from build123d import *

# Parameters (mm, degrees)
Y_KSEKLIK_EKSTR_ZYON1_DEPTH = 12
KES_EKSTR_ZYON1_DEPTH       = 10
KES_EKSTR_ZYON4_DEPTH       = 20
IZIM4_W                     = 6
IZIM4_H                     = 12
Y_KSEKLIK_EKSTR_ZYON2_DEPTH = 30
IZIM5_R                     = 2
KES_EKSTR_ZYON5_DEPTH       = 60


with BuildPart() as part:
    # Çizim1 → Yükseklik-Ekstrüzyon1 (new body)
    with BuildSketch(Plane.XY):
        with BuildLine():
            Line((-2.88077248, -55), (82.297274127, -55))
            ThreePointArc((82.297274127, -55), (131.991875204, 23.567915135), (39.708250823, 34.801940953))
            ThreePointArc((39.708250823, 34.801940953), (-52.575373557, 23.567915135), (-2.88077248, -55))
        make_face()
    extrude(amount=Y_KSEKLIK_EKSTR_ZYON1_DEPTH)

    # Çizim2 → Kes-Ekstrüzyon1 (cut, symmetric)
    with BuildSketch(Plane.XY):
        with BuildLine():
            Line((82.297274127, -53.5), (-2.88077248, -53.5))
            ThreePointArc((-2.88077248, -53.5), (-50.81065631, 23.769228763), (39.708250823, 32.379393047))
            ThreePointArc((39.708250823, 32.379393047), (130.227157957, 23.769228763), (82.297274127, -53.5))
        make_face()
    extrude(amount=KES_EKSTR_ZYON1_DEPTH, both=True, mode=Mode.SUBTRACT)

    # Çizim3 → Kes-Ekstrüzyon4 (cut)
    with BuildSketch(Plane.XZ.offset(55)):
        with BuildLine():
            Line((25.295548254, 4.99642351), (25.295548254, 0))
            Line((25.295548254, 0), (33.431042786, 0))
            Line((33.431042786, 0), (33.431042786, 4.99642351))
            ThreePointArc((33.431042786, 4.99642351), (29.36329552, 9.064170776), (25.295548254, 4.99642351))
        make_face()
        with BuildLine():
            Line((35.422473694, 4.99642351), (35.422473694, 0))
            Line((35.422473694, 0), (43.422473694, 0))
            Line((43.422473694, 0), (43.422473694, 4.99642351))
            ThreePointArc((43.422473694, 4.99642351), (39.422473694, 8.99642351), (35.422473694, 4.99642351))
        make_face()
        with BuildLine():
            Line((45.619413975, 4.99642351), (45.619413975, 0))
            Line((45.619413975, 0), (53.887629124, 0))
            Line((53.887629124, 0), (53.887629124, 4.99642351))
            ThreePointArc((53.887629124, 4.99642351), (49.753521549, 9.130531084), (45.619413975, 4.99642351))
        make_face()
    extrude(amount=-KES_EKSTR_ZYON4_DEPTH, mode=Mode.SUBTRACT)

    # Çizim4 → Yükseklik-Ekstrüzyon2 (add)
    with BuildSketch(Plane(origin=(0, -55, 0), x_dir=(-1, 0, 0), z_dir=(0, -1, 0))):
        with Locations((-17.243778266, -6)):
            Rectangle(IZIM4_W, IZIM4_H)
        with Locations((-61.695384492, -6)):
            Rectangle(IZIM4_W, IZIM4_H)
    extrude(amount=Y_KSEKLIK_EKSTR_ZYON2_DEPTH)

    # Çizim5 → Kes-Ekstrüzyon5 (cut)
    with BuildSketch(Plane(origin=(64.695384492, 0, 0), x_dir=(0, 0, -1), z_dir=(1, 0, 0))):
        with Locations(Location((-6, -81.004647187, 0), (0, 0, 90))):
            Circle(IZIM5_R)
    extrude(amount=-KES_EKSTR_ZYON5_DEPTH, mode=Mode.SUBTRACT)


solid = part.part
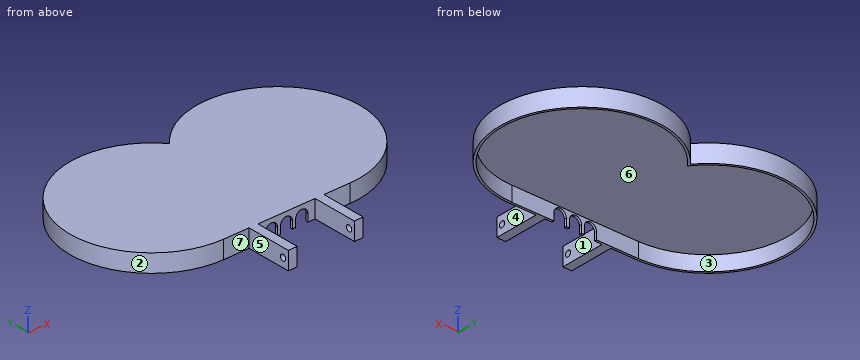
Can you work these out from the model? Positions are in its coordinate system, mm. Face numbers are marked on the shaded views. A direction names the side the tool comes from. Coordinates: 2 decimals unless noted, no trailing zeros. Write each loop counter-clockwise with the first axis right and the second up, starting at its lowest first coordinate (ties: lowest second). Pieces come first, ordered by that corner, then holes. Notation, with made-up numbers: (-36.5, 54.5) -> (-29.5, 54.5) arc R29 cw to (-29.5, 80.5) -> close; hole circle Ø8 at (68, 67.25). An arc over 180 degrees is marked (long way). Write each question's results on one line, items separated by ' | '. Start each with the question number.
Item 1: On a 3-axis mill with a long thin cutter (end or side, diameter ignored), from which of +Z, -Z, +X, -X, +Y, -Y can I reach the whole of each face in a straight line? I mean the marked faces 1, 2 and 3. Say none if no direction works.
Item 2: If we section it at B-B, the plane x = 116.5: Write out the boundary of the cut face in (y, z), and give its area (3 significant figures).
Item 3: Please list where these lines run through material, in increasing order: probe 1 along X at (y, z) = (-56, 1); probe 2 along X at (y, z) = (2, 5.75); probe 3 along X at (y, z) = (40.5, 3.25).
Item 4: Thinking about a two-plate mould opening in X: for the marked faces 4, 5, 6 and 7, which applies, released by +X, released by -X, zero draft, split by the parting line, or undercut?
Item 5: I'm going to push flat-ended pins straight in: P1, Ø5, axis at y = -62, z = 10, coming from the -X side; P2, Ø5, axis at x = 36, z = 6, coming from the +Y side; P3, Ø4, axis at x = 6.5, z = 4, coming from the -Y side. Where does each tip first touch, or does it pass through?
Item 6: If we section it at A-A, the plane y = 0: Write out the boundary of the cut face in (x, z).
Answer block:
1) face 1: +Z, -Z, -Y | face 2: +Z, -Z | face 3: -Z
2) outline: (-43.07, 0) -> (-41.14, 0) -> (-41.14, 10) -> (41.14, 10) -> (41.14, 0) -> (43.07, 0) -> (43.07, 12) -> (-43.07, 12) -> close | area: 211 mm²
3) probe 1: 14.24 to 20.24, 58.7 to 64.7 | probe 2: -57.84 to -56.34, 135.76 to 137.26 | probe 3: -40.09 to -37.84, 32.08 to 34.33, 45.09 to 47.34, 117.25 to 119.51
4) face 4: released by +X | face 5: released by -X | face 6: undercut | face 7: zero draft
5) P1: x = 14.24 | P2: y = 41.25 | P3: y = -55
6) outline: (-57.88, 0) -> (-56.38, 0) -> (-56.38, 10) -> (135.8, 10) -> (135.8, 0) -> (137.3, 0) -> (137.3, 12) -> (-57.88, 12) -> close
